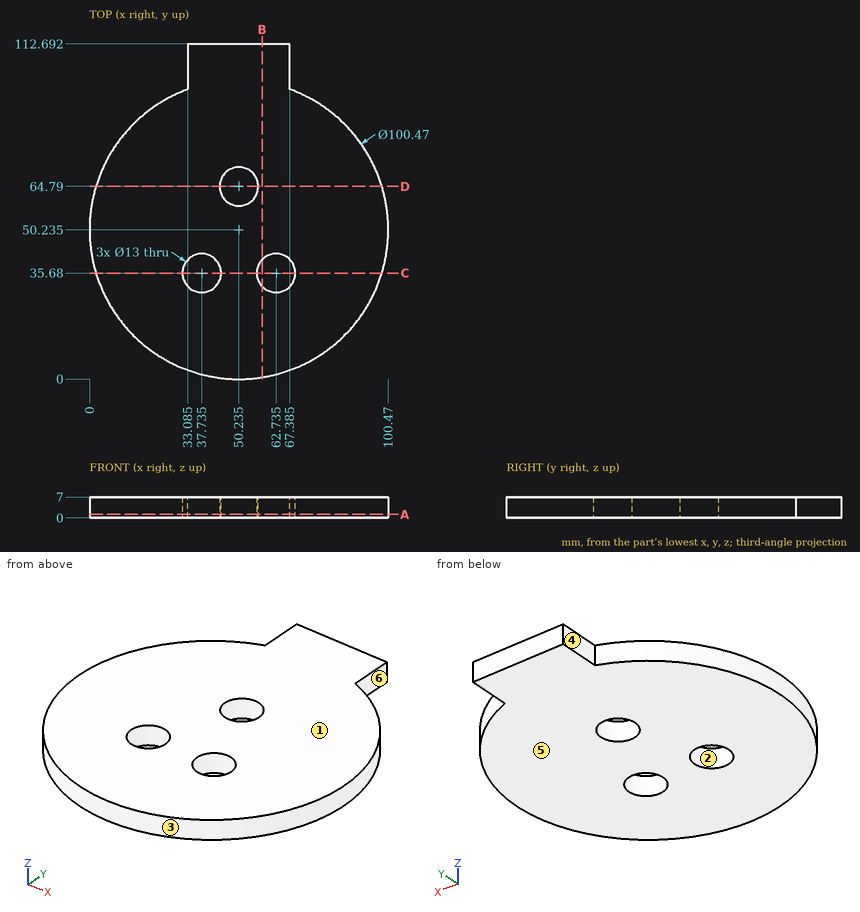
Drawing for the job (mm, zero at the part's lowest x, y, z). A direction names the side the tool comes from. Coordinates: 2 decimals unless noted, no trailing zeros. Write each loop counter-clockwise with the first axis right and the second up, starting at its lowest first coordinate (ties: lowest second). Pieces come first, ordered by that corner, then holes. Notation, with made-up numbers: (8, 52.5) - (28, 52.5) arc R5 cw to (28, 61.5) - close; hole circle Ø1 at (87, -5). An arc over 180 degrees is marked (long way). Write each question's results on one line, items separated by ' | '. Start each with the question number.
1) Cut at A-A (z = 1.25). Write the cut outline in (x, y) (3 decimals).
2) Cut at C-C (y = 35.68). Write the cut outline in (x, z) (3 decimals), then the cut area to 3 significant figures.
3) 3-axis set-ups, long thin cutter, end or side, ignore diameter. For the marked faces 4, 5 and 6: which of +Z, -Z, +X, -X, +Y, -Y reach the whole face in a straight line?
4) Cut at B-B (x = 58). Write the cut outline in (y, z).
5) Cut at D-D (y = 64.79). Write the cut outline in (x, z) (3 decimals), then the cut area to 3 significant figures.
6) Mould opens along Y. For the marked faces 1, 2 and 3 say: pulls with the +Y half, pulls with the -Y half, needs draft (parallel to the pull), parting line crosses it, or undercut.
7) Flat gauge pins, fed straight in: P1, Ø10.5, axis at x = 62.735, y = 35.68, coming from the +Z side; P2, Ø2, axis at x = 81.5, z = 3.5, coming from the +Y side; P3, Ø3.5, axis at y = 107, z = 2.5, coming from the +X side (3 decimals); P4, Ø1, axis at x = 54, z = 3.5, coming from the -Y side. Where does each tip first touch, or does it go through?
8) Probe line 1 along X through (y, z) = (35.5, 6); line 2 along Y through (x, z) = (57.5, 4.5); line 3 along X through (y, z) = (60, 5.5). List the from-to ranges inside material, lowest first. Write a range as from..to.
Returned:
1) outline: (33.085, 97.452) arc R50.235 ccw (long way) to (67.385, 97.452) - (67.385, 112.692) - (33.085, 112.692) - close; hole circle Ø13 at (37.735, 35.68); hole circle Ø13 at (50.235, 64.79); hole circle Ø13 at (62.735, 35.68)
2) outline: (2.155, 0) - (31.235, 0) - (31.235, 7) - (2.155, 7) - close; (44.235, 0) - (56.235, 0) - (56.235, 7) - (44.235, 7) - close; (69.235, 0) - (98.315, 0) - (98.315, 7) - (69.235, 7) - close | area: 491 mm^2
3) face 4: +Z, -Z, -X, +Y | face 5: -Z, +X, -X, +Y, -Y | face 6: +Z, -Z, +X, +Y
4) outline: (0.6, 0) - (31.23, 0) - (31.23, 7) - (0.6, 7) - close; (40.13, 0) - (112.69, 0) - (112.69, 7) - (40.13, 7) - close
5) outline: (2.155, 0) - (43.735, 0) - (43.735, 7) - (2.155, 7) - close; (56.735, 0) - (98.315, 0) - (98.315, 7) - (56.735, 7) - close | area: 582 mm^2
6) face 1: needs draft | face 2: undercut | face 3: parting line crosses it
7) P1: through | P2: y = 90.33 | P3: x = 67.385 | P4: y = 0.11
8) line 1: 2.21..31.24, 44.23..56.24, 69.23..98.26 | line 2: 0.53..31.83, 39.53..112.69 | line 3: 0.96..45.84, 54.63..99.51
